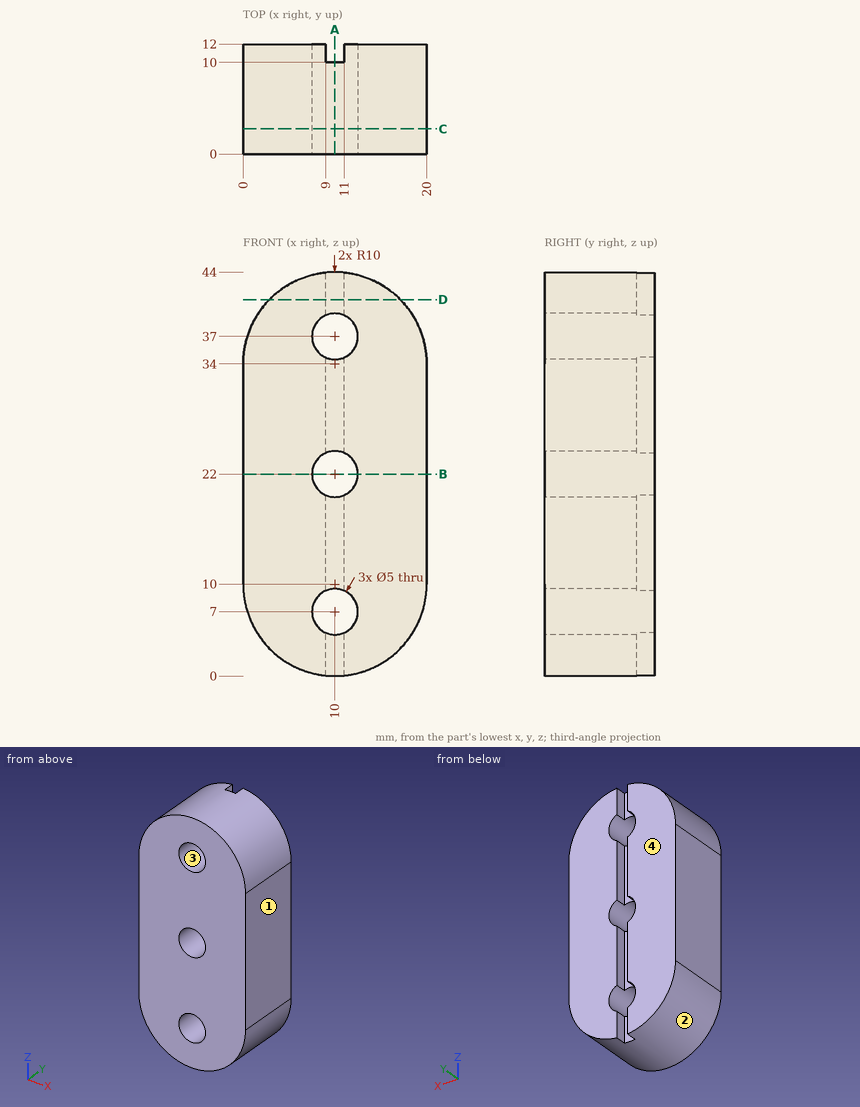
Geometry check sheet. Reference: drawing and pictorial views, mm from the part's lowest x, y, z. Give positions to 0.01 mm unless a question says otherwise; leave off trailing zeros. Order: outer loops, then holes, each group sorted by start corner. A loop starts at its lowest first (then second) coordinate and runs counter-clockwise, first axis right, second up. Notation, with made-up numbers: (88, -22) - (124, -22) arc R25 ccw to (124, -10) - close; hole circle Ø5 at (60, -29). An arc over 180 degrees is marked (long way). Answer as CSV lines item,"result". Start each with the question number.
Item 1: Section check C-C, the plane y = 2.75. Record the boundary of the cut face in (x, z), plus the area to 3 significant figures.
Item 2: Section check A-A, the plane x = 10. Record the boundary of the cut face in (y, z), plus the area to 3 significant figures.
Item 3: Section check D-D, the plane z = 41. Record the boundary of the cut face in (x, y).
Item 4: Material ranges on L1, parallel to Z at x = 10, y = 8; L2, parallel to Z at x = 8.75, y = 6.25; L3, parallel to X at y = 4.25, z = 22, recorded low to high.
Item 5: Mould release check, pull along X, two halves, no side actions. Record for the marked faces 1, 2, 3 and 4: released by +X, released by -X, zero draft, split by the parting line, or undercut.
Item 6: Section check B-B, the plane z = 22. Record the boundary of the cut face in (x, y).
Item 7: Gauge pin test, flat ends, axial feed: pin 1 (1.6 mm diameter, centred on x = 10, z = 1, fed in from +Y); pin 2 (4 mm diameter, centred on x = 10, z = 7, fed in from +Y); pin 3 (0.6 mm diameter, centred on y = 11, z = 41, fed in from +X); pin 4 (1.6 mm diameter, centred on y = 10.5, z = 1.5, fed in from +X). Record the tip position at first contact, or that the pin passes through.
Filled in:
1,outline,"(0, 10) arc R10 ccw to (20, 10) - (20, 34) arc R10 ccw to (0, 34) - close; hole circle Ø5 at (10, 7); hole circle Ø5 at (10, 22); hole circle Ø5 at (10, 37)"
1,area,"735 mm^2"
2,outline,"(0, 0) - (10, 0) - (10, 4.5) - (0, 4.5) - close; (0, 9.5) - (10, 9.5) - (10, 19.5) - (0, 19.5) - close; (0, 24.5) - (10, 24.5) - (10, 34.5) - (0, 34.5) - close; (0, 39.5) - (10, 39.5) - (10, 44) - (0, 44) - close"
2,area,"290 mm^2"
3,outline,"(2.86, 0) - (17.14, 0) - (17.14, 12) - (11, 12) - (11, 10) - (9, 10) - (9, 12) - (2.86, 12) - close"
4,L1,"0 to 4.5, 9.5 to 19.5, 24.5 to 34.5, 39.5 to 44"
4,L2,"0.08 to 4.83, 9.17 to 19.83, 24.17 to 34.83, 39.17 to 43.92"
4,L3,"0 to 7.5, 12.5 to 20"
5,face 1,"released by +X"
5,face 2,"split by the parting line"
5,face 3,"undercut"
5,face 4,"zero draft"
6,outline,"(0, 0) - (7.5, 0) - (7.5, 12) - (0, 12) - close; (12.5, 0) - (20, 0) - (20, 12) - (12.5, 12) - close"
7,pin 1,"y = 10"
7,pin 2,"through"
7,pin 3,"x = 17.42"
7,pin 4,"x = 16.38"
